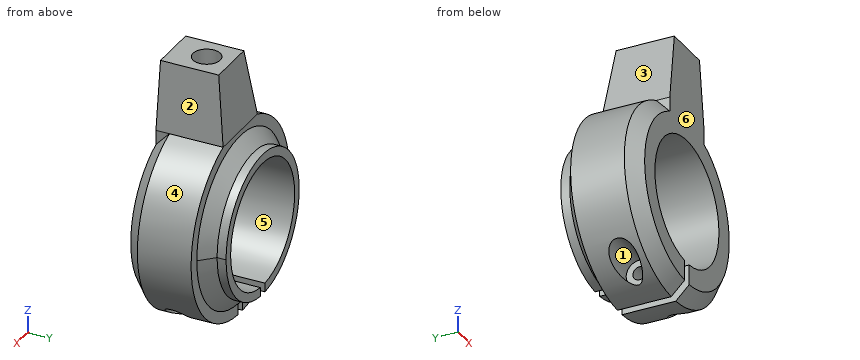
```python
from build123d import *
from OCP.BRepFilletAPI import BRepFilletAPI_MakeChamfer

# Parameters (mm, degrees)
BOSS_EXTRUDE1_DEPTH     = 15
SKETCH2_R               = 3.05
CUT_EXTRUDE1_DEPTH      = 15
BOSS_EXTRUDE2_DEPTH     = 5
CHAMFER4_SIZE           = 3
CHAMFER6_SIZE           = 15
CHAMFER6_SIZE_2         = 2
CUT_EXTRUDE2_DEPTH      = 29
CUT_EXTRUDE2_DEPTH_BACK = 25
SKETCH4_R               = 1.5
SKETCH5_R               = 2.5
CUT_EXTRUDE3_DEPTH      = 20.5
SKETCH6_R               = 3
CUT_EXTRUDE4_DEPTH      = 15.5


with BuildPart() as part:
    # Sketch1 → Boss-Extrude1 (new body)
    with BuildSketch(Plane(origin=(0, 0, 0), x_dir=(1, 0, 0), z_dir=(0, 1, 0))):
        with BuildLine():
            ThreePointArc((-14.719179189, 17.95673597), (-15.719179189, -10.007504074), (-16.719179189, 17.95673597))
            Line((-16.719179189, 17.95673597), (-16.719179189, 25.469227521))
            ThreePointArc((-16.719179189, 25.469227521), (-36.961756137, 7.309561592), (-23.219179189, -16.156945753))
            Line((-23.219179189, -16.156945753), (-23.219179189, -31.156945753))
            Line((-23.219179189, -31.156945753), (-8.219179189, -31.156945753))
            Line((-8.219179189, -31.156945753), (-8.219179189, -16.156945753))
            ThreePointArc((-8.219179189, -16.156945753), (5.523397758, 7.309561592), (-14.719179189, 25.469227521))
            Line((-14.719179189, 25.469227521), (-14.719179189, 17.95673597))
        make_face()
    extrude(amount=BOSS_EXTRUDE1_DEPTH)

    # Sketch2 → Cut-Extrude1 (cut)
    with BuildSketch(Plane.XY.offset(31.156945753)):
        with Locations((-15.719179189, 7.5)):
            Circle(SKETCH2_R)
    extrude(amount=-CUT_EXTRUDE1_DEPTH, mode=Mode.SUBTRACT)

    # Sketch3 → Boss-Extrude2 (add)
    with BuildSketch(Plane(origin=(0, 15, 0), x_dir=(1, 0, 0), z_dir=(0, 1, 0))):
        with BuildLine():
            Line((-16.719179189, 17.95673597), (-16.719179189, 19.961215349))
            ThreePointArc((-16.719179189, 19.961215349), (-26.673630339, -7.669407863), (0.280820811, 3.992495926))
            ThreePointArc((0.280820811, 3.992495926), (-4.0572754, 14.946947076), (-14.719179189, 19.961215349))
            Line((-14.719179189, 19.961215349), (-14.719179189, 17.95673597))
            ThreePointArc((-14.719179189, 17.95673597), (-15.719179189, -10.007504074), (-16.719179189, 17.95673597))
        make_face()
    extrude(amount=BOSS_EXTRUDE2_DEPTH)

    # Chamfer4
    chamfer4_edges = [part.edges().sort_by_distance(p)[0] for p in [
        (-26.673630339, 15, 7.669407863),
        (-36.961756137, 0, -7.309561592),
        (5.523397758, 0, -7.309561592),
    ]]
    chamfer(chamfer4_edges, length=CHAMFER4_SIZE)

    # Chamfer6
    chamfer6_edges_1 = [part.edges().sort_by_distance(p)[0] for p in [
        (-23.219179189, 7.5, 31.156945753),
    ]]
    chamfer6_side_1 = [part.faces().sort_by_distance(p)[0] for p in [
        (-23.219179189, 7.5, 31.116945753),
    ]]
    chamfer6_edges_2 = [part.edges().sort_by_distance(p)[0] for p in [
        (-8.219179189, 7.5, 31.156945753),
    ]]
    chamfer6_side_2 = [part.faces().sort_by_distance(p)[0] for p in [
        (-8.259179189, 7.5, 31.156945753),
    ]]
    chamfer6_edges_3 = [part.edges().sort_by_distance(p)[0] for p in [
        (-15.719179189, 15, 31.156945753),
    ]]
    chamfer6_side_3 = [part.faces().sort_by_distance(p)[0] for p in [
        (-15.719179189, 14.96, 31.156945753),
    ]]
    chamfer6 = BRepFilletAPI_MakeChamfer(part.part.solid().wrapped)
    for e in chamfer6_edges_1:
        chamfer6.Add(CHAMFER6_SIZE - 0.0001, CHAMFER6_SIZE_2 - 0.0001, e.wrapped, chamfer6_side_1[0].wrapped)
    for e in chamfer6_edges_2:
        chamfer6.Add(CHAMFER6_SIZE_2 - 0.0001, CHAMFER6_SIZE - 0.0001, e.wrapped, chamfer6_side_2[0].wrapped)
    for e in chamfer6_edges_3:
        chamfer6.Add(CHAMFER6_SIZE_2 - 0.0001, CHAMFER6_SIZE - 0.0001, e.wrapped, chamfer6_side_3[0].wrapped)
    add(Compound.cast(chamfer6.Shape()), mode=Mode.REPLACE)  # a hair under: the kernel refuses the full size

    # Sketch4 → Cut-Extrude2 (cut, two sides: drawn at the far end of the back side and taken through both)
    with BuildSketch(Plane.ZY.offset(14.719179189).offset(-CUT_EXTRUDE2_DEPTH_BACK)):
        with Locations(Location((-21.469227521, 7.5, 0), (0, 0, 180))):
            Circle(SKETCH4_R)
    extrude(amount=CUT_EXTRUDE2_DEPTH + CUT_EXTRUDE2_DEPTH_BACK, mode=Mode.SUBTRACT)

    # Sketch5 → Cut-Extrude3 (cut)
    with BuildSketch(Plane(origin=(5.780820811, 0, 0), x_dir=(0, 0, -1), z_dir=(1, 0, 0))):
        with Locations((21.469227521, 7.5)):
            Circle(SKETCH5_R)
    extrude(amount=-CUT_EXTRUDE3_DEPTH, mode=Mode.SUBTRACT)

    # Sketch6 → Cut-Extrude4 (cut)
    with BuildSketch(Plane.ZY.offset(37.219179189)):
        with Locations((-21.469227521, 7.5)):
            Circle(SKETCH6_R)
    extrude(amount=-CUT_EXTRUDE4_DEPTH, mode=Mode.SUBTRACT)


solid = part.part
```
Work out the finished part from the listing and answer in its coordinate system (mm). Face numbers are marked on the shaded views. A direction names the side the tool comes from. Give positions to 0.01 mm unless a question says otherwise; leave off trailing zeros. Write each loop counter-clockwise with the first axis right and the second up, starting at its lowest first coordinate (ties: lowest second). Pieces come first, ordered by that corner, then holes. Notation, with made-up numbers: (52, 68.25) -> (76, 68.25) arc R12 ccw to (76, 72.25) -> close; hole circle Ø9 at (-31, 75). An arc over 180 degrees is marked (long way). Write each question's results on one line, items separated by ' | '.
1. Find section B-B on z = 25. Determine the outline of the cut face in (x, y), and give its area (4 significant figures).
Data:
outline: (-22.04, 0) -> (-9.4, 0) -> (-9.4, 13.82) -> (-22.04, 13.82) -> close; hole circle Ø6.1 at (-15.72, 7.5) | area: 145.5 mm^2
2. Straight lines are drawn through the part: L1, parallel to X at y = 12, z = -4.5; L2, parallel to X at y = 11.25, z = 4; L3, parallel to Z at x = -19.5, y = 4.5. For each, find the intervals that lie inside material, in ascending order.
Data:
L1: -37.21 to -29.71, -1.73 to 5.77 | L2: -35.68 to -27.21, -4.22 to 4.24 | L3: -25.16 to -17.47, 9.49 to 31.16
3. Find section A-A on y = 7.5. Give the number of separate pieces and of enclosed holes in the cut face, and give its area (3 significant figures).
Data:
separate pieces: 3 | enclosed holes: 0 | area: 803 mm^2
4. Each of these flat-tipped pins is pushed along its axis until it touches: pin 1 Ø4 at (y, z) = (7.5, -21.47) entering from +X; pin 2 Ø2.5 at (y, z) = (5, -20.5) entering from -X; pin 3 Ø1 at (y, z) = (7.5, 15) entering from -X; pin 4 Ø25 at (x, z) = (-15.72, -3.99) entering from +Y. Where does it stop, or does it pass through?
Data:
pin 1: x = -16.72 | pin 2: x = -30.87 | pin 3: x = -26.69 | pin 4: through
5. Determine the mould class of the marked faces 3, 4, 5 and 6 for opening direction Z: +Z half, -Z half, draft (parallel to the pull), parting line (faces both ways), or undercut.
Data:
face 3: +Z half | face 4: parting line | face 5: undercut | face 6: draft
6. A tool of negligible diameter and unlimited length cuts with its end or side. For the marked faces 1 and 2, from which of +Z, -Z, +X, -X, +Y, -Y can it reach the whole face along a straight path? Write none if from no direction.
Data:
face 1: -X | face 2: +Z, +X, +Y, -Y
7. Find section C-C on y = 1.75. Determine the outline of the cut face in (x, z).
Data:
outline: (-23.22, 14.82) arc R20.25 ccw to (-16.72, -24.22) -> (-16.72, -17.96) arc R14 cw (long way) to (-14.72, -17.96) -> (-14.72, -24.22) arc R20.25 ccw to (-8.22, 14.82) -> (-8.22, 16.16) -> (-10.22, 31.16) -> (-21.22, 31.16) -> (-23.22, 16.16) -> close
